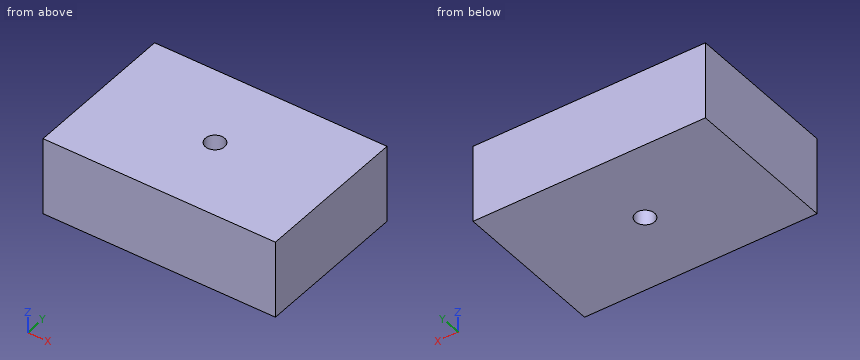
```python
from build123d import *

# Parameters (mm, degrees)
F0_W     = 101.6
F0_H     = 50.8
F1_DEPTH = 152.4
F2_R     = 6.35
F3_DEPTH = 50.8


with BuildPart() as f1:
    # F0 (on Right) → F1 (new body)
    with BuildSketch(Plane.YZ):
        with Locations((50.8, 25.4)):
            Rectangle(F0_W, F0_H)
    extrude(amount=F1_DEPTH)

    # F2 (on face) → F3 (cut)
    with BuildSketch(Plane(origin=(0, 0, 0), x_dir=(1, 0, 0), z_dir=(0, 0, -1))):
        with Locations((76.2, -50.8)):
            Circle(F2_R)
    extrude(amount=-F3_DEPTH, mode=Mode.SUBTRACT)


solid = f1.part
```
Here's how the part is built. I have some questions about the finished solid (model axes, mm). Round coordinates to 2 decimals unless told otherwise and drop trailing zeros. Write each loop counter-clockwise with the first axis right and the second up, starting at its lowest first coordinate (ties: lowest second). Pieces come first, ordered by that corner, then holes.
Q1. Please list where these lines run through material, in increasing order: probe 1 along Y at (x, z) = (76, 40); probe 2 along X at (y, z) = (50.8, 36); probe 3 along X at (y, z) = (55, 24).
Q2. If we section it at B-B on x = 76.2: Write out the boundary of the cut face in (y, z).
Q3. If we section it at A-A on y = 50.8: Write out the boundary of the cut face in (x, z).
Answer below:
1. probe 1: y = 0 to 44.45, 57.15 to 101.6
1. probe 2: x = 0 to 69.85, 82.55 to 152.4
1. probe 3: x = 0 to 71.44, 80.96 to 152.4
2. outline: (0, 0) - (44.45, 0) - (44.45, 50.8) - (0, 50.8) - close; (57.15, 0) - (101.6, 0) - (101.6, 50.8) - (57.15, 50.8) - close
3. outline: (0, 0) - (69.85, 0) - (69.85, 50.8) - (0, 50.8) - close; (82.55, 0) - (152.4, 0) - (152.4, 50.8) - (82.55, 50.8) - close
